from build123d import *

# Parameters (mm, degrees)
F1_DEPTH = 63.5
F0_W     = 25.4
F0_H     = 19.05
F2_DEPTH = 25.4
F3_DEPTH = 7.9375
F5_R     = 6.35


# Not quite as in the source:
# - a feature names something its author has since deleted; it is built from what else it names


with BuildPart() as f1:
    # F0 (on Front) → F1 (new body, symmetric)
    with BuildSketch(Plane.XZ):
        Polygon((41.275, -9.525), (41.275, 9.525), (22.225, 9.525), (-41.275, 9.525), (-41.275, -9.525), align=None)
    extrude(amount=F1_DEPTH, both=True)

    # F0 (on Front) → F2 (join, symmetric)
    with BuildSketch(Plane.XZ):
        with BuildLine():
            Line((22.225, 9.525), (41.275, 9.525))
            Line((41.275, 9.525), (41.275, 27.0002))
            ThreePointArc((41.275, 27.0002), (45.9246798487, 38.2255201513), (57.15, 42.8752))
            Line((57.15, 42.8752), (60.325, 42.8752))
            Line((60.325, 42.8752), (60.325, 61.9252))
            Line((60.325, 61.9252), (57.15, 61.9252))
            add(Edge.make_bspline(
                [(49.7646190409, 61.1353984481), (52.2104568014, 61.4669327128), (54.6731104701, 61.7311893911), (57.15, 61.9252)],
                knots=[104.645371818, 104.645371818, 104.645371818, 104.645371818, 111.5045361635, 111.5045361635, 111.5045361635, 111.5045361635], degree=3))
            ThreePointArc((49.7646190409, 61.1353984481), (29.9682960891, 48.9298739032), (22.225, 27.0002))
            Line((22.225, 27.0002), (22.225, 9.525))
        make_face()
        with Locations((73.025, 52.4002)):
            Rectangle(F0_W, F0_H)
    extrude(amount=F2_DEPTH, both=True)

    # F0 (on Front) → F3 (join, symmetric)
    with BuildSketch(Plane.XZ):
        with BuildLine():
            Line((-41.275, 9.525), (22.225, 9.525))
            Line((22.225, 9.525), (22.225, 27.0002))
            ThreePointArc((22.225, 27.0002), (29.9682960891, 48.9298739032), (49.7646190409, 61.1353984481))
            add(Edge.make_bspline(
                [(-41.275, 9.525), (-20.9502066659, 35.3602907495), (12.4502190704, 56.0774169419), (49.7646190409, 61.1353984481)],
                knots=[0, 0, 0, 0, 104.645371818, 104.645371818, 104.645371818, 104.645371818], degree=3))
        make_face()
    extrude(amount=F3_DEPTH, both=True)

    # F0 (on Front) → F4 (revolve)
    with BuildSketch(Plane.XZ):
        Polygon((85.725, 61.9252), (85.725, 42.8752), (85.725, 38.1), (111.125, 38.1), (111.125, 66.675), (85.725, 66.675), align=None)
    revolve(axis=Axis((85.725, 0, 52.3875), (0, 0, 1)))

    # F5
    f5_edges = [f1.edges().sort_by_distance(p)[0] for p in [
        (41.275, -63.5, 0),
        (41.275, 63.5, 0),
        (-41.275, 63.5, 0),
        (-41.275, -63.5, 0),
    ]]
    fillet(f5_edges, radius=F5_R)


solid = f1.part
Design review of the part built by this model. Coordinates are the model's own, in mm. A direction names the side the tool comes from. Coordinates: 2 decimals unless noted, no trailing zeros. Loops run counter-clockwise (first coordinate to the right, second up) from the corner with the lowest first, then second, coordinate; pieces in that order, holes last. Notation, with made-up numbers: M 42,56.5 L 62,56.5 A21 ccw 62,69.5 Z; hole C 18,89.25 d8. An arc over 180 degrees is marked long. Use one line per item in the form item = value.
(1) Clearance check with flat-ended pins moving along their axes: P1, Ø10, axis at x = -0.5, y = -9.5, coming from the +Z side; P2, Ø5, axis at x = 58, y = 0, coming from the -Z side; P3, Ø14, axis at y = 16.5, z = 17, coming from the -X side (3 decimals). State where each tip first meets the part, or that it passes through.
Return value:
P1 = 46.62
P2 = 38.1
P3 = 22.225
(2) Consider section A-A (z = 2). Write out the cut boundary in (x, y) (3 decimals), and give its area (3 significant figures).
Return value:
outline = M -41.275,-57.15 A6.35 ccw -34.925,-63.5 L 34.925,-63.5 A6.35 ccw 41.275,-57.15 L 41.275,57.15 A6.35 ccw 34.925,63.5 L -34.925,63.5 A6.35 ccw -41.275,57.15 Z
area = 10,400 mm2
(3) For line 1 along X through (y, z) = (47, 6.5) (3 decimals); line 2 along Z through (x, y) = (80.5, -25); line 3 along Z through (x, y) = (9, -13.5) (3 decimals), list the stretches that pass through material, from the lowest coordinate up. Write a range as from..to.
Return value:
line_1 = -41.275..41.275
line_2 = 42.88..61.93
line_3 = -9.525..9.525
(4) Consider section B-B (x = 64.5). Write out the cut boundary in (y, z) (3 decimals).
Return value:
outline = M -25.4,42.875 L -13.952,42.875 L -13.952,38.1 L 13.952,38.1 L 13.952,42.875 L 25.4,42.875 L 25.4,61.925 L 13.952,61.925 L 13.952,66.675 L -13.952,66.675 L -13.952,61.925 L -25.4,61.925 Z
(5) For faces 1 (the face through (60, -2, 61.925)), 2 (the face through (41.275, -1, 4)), 3 (the face through (22.225, -17, 18)), 4 (the face through (46, 25.4, 42)), 5 (the face through (1, 35, 9.525)), list the 3-axis set-ups (+Z, -Z, +X, -X, +Y, -Y) from which the entire face can be reached by the end or side of a thin tool; tool diameter is ignored.
Return value:
face_1 = +Z, -X
face_2 = -Z, +X, +Y, -Y
face_3 = +Z, -X, -Y
face_4 = +Z, +X, -X, +Y
face_5 = +Z, -X, +Y
(6) Draft analysis for pull direction X (two halves, no side actions). For faces 6 (the face through (0, 63.5, 0)), 7 (the face through (30.18, -16.79, 49.19)), 8 (the face through (60, 2, 42.875)), state which applies: pulls with the +X half, pulls with the -X half, needs draft (parallel to the pull), parting line crosses it, or undercut.
Return value:
face_6 = needs draft
face_7 = pulls with the -X half
face_8 = undercut
